Source: CAD feature listing. Evaluate the final solid. Frame: model axes, mm. A direction names the side the tool comes from. Round coordinates to 2 decimals unless told otherwise and drop trailing zeros. Loops run counter-clockwise (first coordinate to the right, second up) from the corner with the lowest first, then second, coordinate; pieces in that order, holes last. Notation, with made-up numbers: M 56,35 L 106,35 A28 cw 106,64 Z; hole C 37.5,-20.75 d6. An arc over 180 degrees is marked long. One line per item, written item: value.
from build123d import *

# Parameters (mm, degrees)
SKETCH2_R              = 3
SKETCH2_R_2            = 3.25
SKETCH2_R_3            = 3.5
MAINPLATEEXTRUDE_DEPTH = 4
SKETCH3_W              = 21
SKETCH3_H              = 4
TOPBEARING_DEPTH       = 12
FILLET1_R              = 10
TOPBEARINGCUT_REACH    = 101.107
SKETCH4_R              = 3


with BuildPart() as part:
    # Sketch2 → MainPlateExtrude (new body)
    with BuildSketch(Plane(origin=(0, 0, 0), x_dir=(1, 0, 0), z_dir=(0, 1, 0))):
        with BuildLine():
            Line((-81.215970545, -46.28367362), (-81.215970545, -16.925572983))
            ThreePointArc((-81.215970545, -16.925572983), (-79.384065752, -11.156498475), (-74.559526408, -7.501103014))
            Line((-74.559526408, -7.501103014), (-8.731304339, 15.853031333))
            ThreePointArc((-8.731304339, 15.853031333), (-3.715970545, 16.71632638), (1.299363248, 15.853031333))
            Line((1.299363248, 15.853031333), (67.127585317, -7.501103014))
            ThreePointArc((67.127585317, -7.501103014), (71.952124662, -11.156498475), (73.784029455, -16.925572983))
            Line((73.784029455, -16.925572983), (73.784029455, -46.28367362))
            ThreePointArc((73.784029455, -46.28367362), (69.390631173, -56.890275338), (58.784029455, -61.28367362))
            add(Edge.make_bspline(
                [(58.784029455, -61.28367362), (24.556467528, -64.469839896), (8.784029455, -84.862635588)],
                knots=[0, 0, 0, 0.615675344, 0.615675344, 0.615675344], degree=2))
            Line((8.784029455, -84.862635588), (-16.215970545, -84.862635588))
            add(Edge.make_bspline(
                [(-66.215970545, -61.28367362), (-31.988408619, -64.469839896), (-16.215970545, -84.862635588)],
                knots=[0, 0, 0, 0.615675344, 0.615675344, 0.615675344], degree=2))
            ThreePointArc((-66.215970545, -61.28367362), (-76.822572263, -56.890275338), (-81.215970545, -46.28367362))
        make_face()
        with Locations(Location((-66.215970545, -46.28367362, 0), (0, 0, 270))):
            Circle(SKETCH2_R, mode=Mode.SUBTRACT)
        with Locations(Location((58.784029455, -46.28367362, 0), (0, 0, 270))):
            Circle(SKETCH2_R, mode=Mode.SUBTRACT)
        with Locations(Location((-3.715970545, -22.362635588, 0), (0, 0, 270))):
            Circle(SKETCH2_R_2, mode=Mode.SUBTRACT)
        with Locations(Location((-3.715970545, -46.28367362, 0), (0, 0, 270))):
            Circle(SKETCH2_R_3, mode=Mode.SUBTRACT)
        with Locations(Location((-3.715970545, -72.362635588, 0), (0, 0, 270))):
            Circle(SKETCH2_R_3, mode=Mode.SUBTRACT)
        with BuildLine():
            Line((-74.215970545, -18.362635588), (-53.215970545, -18.362635588))
            ThreePointArc((-53.215970545, -18.362635588), (-51.801756983, -18.948422026), (-51.215970545, -20.362635588))
            Line((-51.215970545, -20.362635588), (-51.215970545, -24.362635588))
            ThreePointArc((-51.215970545, -24.362635588), (-51.801756983, -25.77684915), (-53.215970545, -26.362635588))
            Line((-53.215970545, -26.362635588), (-74.215970545, -26.362635588))
            ThreePointArc((-74.215970545, -26.362635588), (-75.630184108, -25.77684915), (-76.215970545, -24.362635588))
            Line((-76.215970545, -24.362635588), (-76.215970545, -20.362635588))
            ThreePointArc((-76.215970545, -20.362635588), (-75.630184108, -18.948422026), (-74.215970545, -18.362635588))
        make_face(mode=Mode.SUBTRACT)
        with BuildLine():
            Line((66.784029455, -26.362635588), (45.784029455, -26.362635588))
            ThreePointArc((45.784029455, -26.362635588), (44.369815892, -25.77684915), (43.784029455, -24.362635588))
            Line((43.784029455, -24.362635588), (43.784029455, -20.362635588))
            ThreePointArc((43.784029455, -20.362635588), (44.369815892, -18.948422026), (45.784029455, -18.362635588))
            Line((45.784029455, -18.362635588), (66.784029455, -18.362635588))
            ThreePointArc((66.784029455, -18.362635588), (68.198243017, -18.948422026), (68.784029455, -20.362635588))
            Line((68.784029455, -20.362635588), (68.784029455, -24.362635588))
            ThreePointArc((68.784029455, -24.362635588), (68.198243017, -25.77684915), (66.784029455, -26.362635588))
        make_face(mode=Mode.SUBTRACT)
        with BuildLine():
            Line((-0.715970545, 4.21632638), (-0.715970545, -0.78367362))
            ThreePointArc((-0.715970545, -0.78367362), (-3.715970545, -3.78367362), (-6.715970545, -0.78367362))
            Line((-6.715970545, -0.78367362), (-6.715970545, 4.21632638))
            ThreePointArc((-6.715970545, 4.21632638), (-3.715970545, 7.21632638), (-0.715970545, 4.21632638))
        make_face(mode=Mode.SUBTRACT)
    extrude(amount=MAINPLATEEXTRUDE_DEPTH)

    # Sketch3 → TopBearing (add)
    with BuildSketch(Plane(origin=(0, 4, 0), x_dir=(1, 0, 0), z_dir=(0, 1, 0))):
        with Locations((-63.715970545, -16.362635588)):
            Rectangle(SKETCH3_W, SKETCH3_H)
        with Locations((-63.715970545, -28.362635588)):
            Rectangle(SKETCH3_W, SKETCH3_H)
        with Locations((56.284029455, -28.362635588)):
            Rectangle(SKETCH3_W, SKETCH3_H)
        with Locations((56.284029455, -16.362635588)):
            Rectangle(SKETCH3_W, SKETCH3_H)
    extrude(amount=TOPBEARING_DEPTH)

    # Fillet1
    fillet1_edges = [part.edges().sort_by_distance(p)[0] for p in [
        (-74.215970545, 16, 16.362635588),
        (-53.215970545, 16, 16.362635588),
        (-74.215970545, 16, 28.362635588),
        (-53.215970545, 16, 28.362635588),
        (45.784029455, 16, 28.362635588),
        (66.784029455, 16, 28.362635588),
        (66.784029455, 16, 16.362635588),
        (45.784029455, 16, 16.362635588),
    ]]
    fillet(fillet1_edges, radius=FILLET1_R)

    # TopBearingCut: up to this face of the body (flat: up to its plane)
    topbearingcut_end = Plane(part.part.faces().sort_by_distance((-63.715970545, 9.226840692, 14.362635588))[0])
    # Sketch4 → TopBearingCut (cut, up to the picked face)
    with BuildSketch(Plane.XY.offset(30.362635588), mode=Mode.PRIVATE) as topbearingcut_sk1:
        with Locations((-63.715970545, 7.927390452)):
            Circle(SKETCH4_R)
    topbearingcut_tool1 = split(extrude(topbearingcut_sk1.sketch, amount=-TOPBEARINGCUT_REACH, mode=Mode.PRIVATE), bisect_by=topbearingcut_end, keep=Keep.BOTH, mode=Mode.PRIVATE)
    # Sketch4 → TopBearingCut (cut, up to the picked face)
    with BuildSketch(Plane.XY.offset(30.362635588), mode=Mode.PRIVATE) as topbearingcut_sk2:
        with Locations((56.284029455, 7.927390452)):
            Circle(SKETCH4_R)
    topbearingcut_tool2 = split(extrude(topbearingcut_sk2.sketch, amount=-TOPBEARINGCUT_REACH, mode=Mode.PRIVATE), bisect_by=topbearingcut_end, keep=Keep.BOTH, mode=Mode.PRIVATE)
    add(topbearingcut_tool1.solids().sort_by(Axis((-63.715971, 7.92739, 30.362636), (0, 0, -1)))[0], mode=Mode.SUBTRACT)
    add(topbearingcut_tool2.solids().sort_by(Axis((56.284029, 7.92739, 30.362636), (0, 0, -1)))[0], mode=Mode.SUBTRACT)


solid = part.part
1. Pin query (flat end, axial travel): pin 1 (3 mm diameter, centred on y = 13, z = 30, fed in from +X); pin 2 (4 mm diameter, centred on y = 13, z = 31.5, fed in from +X); pin 3 (5 mm diameter, centred on x = -54, y = 6, fed in from -Z); pin 4 (6 mm diameter, centred on y = 5.5, z = 32, fed in from -X). Return the tip coordinate at first contact, or that it passes through.
Report:
pin 1: stops at x = 65.14
pin 2: stops at x = 65.23
pin 3: stops at z = -0.33
pin 4: stops at x = -81.22
2. Reachability of faces 1 (the face through (48.636, 12.993, 16.335)), 2 (the face through (43.784, 2, 22)), 3 (the face through (63.932, 12.993, 16.335)), 4 (the face through (-63.9, 11.2, 30.363)), 5 (the face through (59.055, 6.778, 28.391)) from +Z, -Z, +X, -X, +Y, -Y: full face, straight path, thin tool, end or side. Return the list, or none.
Report:
face 1: +Z, -Z, +Y
face 2: +Y, -Y
face 3: +Z, -Z, +X, +Y
face 4: +Z, +X, -X, +Y
face 5: +Z, -Z
3. Section query A-A (y = 13). Return the cut outline in (x, z).
Report:
outline: M -71.36,14.36 L -56.07,14.36 L -56.07,18.36 L -71.36,18.36 Z; M -71.36,26.36 L -56.07,26.36 L -56.07,30.36 L -71.36,30.36 Z; M 48.64,14.36 L 63.93,14.36 L 63.93,18.36 L 48.64,18.36 Z; M 48.64,26.36 L 63.93,26.36 L 63.93,30.36 L 48.64,30.36 Z
4. Section query C-C (z = -10). Return the cut outline in (x, y).
Report:
outline: M -25.23,0 L 17.8,0 L 17.8,4 L -25.23,4 Z
5. Ray query, line 1 (Z direction, x = 50, y = 5.5); line 2 (Y direction, x = 21, z = 50.5); line 3 (Z direction, x = -55.5, y = 1). Return the intervals inside material, ascending. Write a range as [from, to].
Report:
line 1: z = [14.36, 18.36], [26.36, 30.36]
line 2: y = [0, 4]
line 3: z = [0.74, 18.36], [26.36, 62.79]
6. Pull-direction query (Z, two-part tool) for faces 6 (the face through (-76.216, 2, 22)), 7 (the face through (-3, 0, 33)), 8 (the face through (-42.11, 1.97, -4.01)); classes: released by +Z, released by -Z, zero draft, split by the parting line, or undercut.
Report:
face 6: undercut
face 7: zero draft
face 8: released by -Z
7. Section query B-B (x = 6). Return the cut outline in (y, z), and give its area (3 significant figures).
Report:
outline: M 0,-14.19 L 4,-14.19 L 4,84.86 L 0,84.86 Z
area: 396 mm2
